Could you check a few things on this model? Use its own coordinates, in mm. A direction names the side the tool comes from. Coordinates: 2 decimals unless noted, no trailing zeros. Write each loop counter-clockwise with the first axis right and the second up, starting at its lowest first coordinate (ties: lowest second). Pieces come first, ordered by that corner, then holes.
```python
from build123d import *

# Parameters (mm, degrees)
F0_R     = 12.7
F1_DEPTH = 152.4
F4_DEPTH = 3.175
F5_SIZE  = 0.762
F6_SIZE  = 0.762


# Not quite as in the source:
# - a pattern or mirror of a feature is missing from the dataset's text; its kind, count and spacing are read off the source's solid


with BuildPart() as f1:
    # F0 (on Front) → F1 (new body, symmetric)
    with BuildSketch(Plane.XZ):
        Circle(F0_R)
    extrude(amount=F1_DEPTH, both=True)

    # F3 (on offset) → F4 (cut)
    with BuildSketch(Plane.XY.offset(12.7)):
        with BuildLine():
            Line((3.175, -156.7815), (3.175, -114.3))
            ThreePointArc((3.175, -114.3), (0, -111.125), (-3.175, -114.3))
            Line((-3.175, -114.3), (-3.175, -156.7815))
            Line((-3.175, -156.7815), (3.175, -156.7815))
        make_face()
    f4 = extrude(amount=-F4_DEPTH, mode=Mode.SUBTRACT)

    # F4_copies: F4 across plane
    add(f4.mirror(Plane.ZX), mode=Mode.SUBTRACT)

    # F5
    f5_edges = [f1.edges().sort_by_distance(p)[0] for p in [
        (-7.77713, -152.4, -10.040232),
    ]]
    chamfer(f5_edges, length=F5_SIZE)

    # F6
    f6_edges = [f1.edges().sort_by_distance(p)[0] for p in [
        (-7.77713, 152.4, -10.040232),
        (10.040232, 152.4, 7.77713),
    ]]
    chamfer(f6_edges, length=F6_SIZE)


solid = f1.part
```
1. For pin 1 (8 mm diameter, centred on x = -6, y = -77, fed in from +Z); pin 2 (3 mm diameter, centred on x = -1.5, y = -133.5, fed in from +Z) (3 decimals); pin 3 (12 mm diameter, centred on x = 7, y = -87.5, fed in from +Z), each with a flat end and sliding along its axis, tell me the tip position at first contact or that it passes through.
Verdict:
pin 1: stops at z = 12.54
pin 2: stops at z = 9.525
pin 3: stops at z = 12.66
2. I want a section at B-B on y = -122. Please give me the cut outline in (x, z) (3 decimals), plus the area to 3 significant figures.
Verdict:
outline: (-3.175, 9.525) - (-3.175, 12.297) arc R12.7 ccw (long way) to (3.175, 12.297) - (3.175, 9.525) - close
area: 487 mm2
3. I want a section at C-C on y = 56.5. Please give me the cut outline in (x, z), plus the area to 3 significant figures.
Verdict:
outline: circle Ø25.4 at (0, 0)
area: 507 mm2
4. Please list where these lines run through material, in increasing order: line 1 along Z through (x, y) = (4.25, 135); line 2 along X through (y, z) = (43.5, -0.25); line 3 along X through (y, z) = (117, 8).
Verdict:
line 1: z = -11.97 to 11.97
line 2: x = -12.7 to 12.7
line 3: x = -9.86 to 9.86
5. If we mould it in two halves opening along X, with no side actions, what happens to faces 1 (the face through (0, 131, 9.525)), 2 (the face through (0, 152.4, 0)), 3 (the face through (-2.75, -2.12, -12.4))? For each: pulls with the +X half, pulls with the -X half, needs draft (parallel to the pull), parting line crosses it, or undercut.
Verdict:
face 1: undercut
face 2: needs draft
face 3: parting line crosses it
6. On a 3-axis mill with a long thin cutter (end or side, diameter ignored), from which of +Z, -Z, +X, -X, +Y, -Y can I reach the whole of each face in a straight line? I mean faces 4 (the face through (0, -152.4, 0)), 5 (the face through (0, -131, 9.525)). Say none if no direction works.
Verdict:
face 4: +Z, -Z, +X, -X, -Y
face 5: +Z, -Y
7. I want a section at A-A on x = 0. Please give me the cut outline in (y, z) (3 decimals).
Verdict:
outline: (-152.4, -11.938) - (-151.638, -12.7) - (151.638, -12.7) - (152.4, -11.938) - (152.4, 9.525) - (111.125, 9.525) - (111.125, 12.7) - (-111.125, 12.7) - (-111.125, 9.525) - (-152.4, 9.525) - close
